For this review, take the finished solid that the model builds, in its own axes (mm). A direction names the side the tool comes from. Coordinates: 2 decimals unless noted, no trailing zeros. Return JSON: item names as keys, results as strings. Group by question number.
Item 1: For line 1 along X through (y, z) = (2, 4.5); line 2 along Y through (x, z) = (8.5, 15); line 3 along Y through (x, z) = (-28, 2.5), list the stretches that pass through material, from the lowest coordinate up.
Item 2: Machinability: for faces 1 (the flat face through (0, 1, 25)), 2 (the cylindrical face through (12.92, 1.24, 23.03)), which of the approach directions +Z, -Z, +X, -X, +Y, -Y give a long, thin tool a straight path to every point of the face, cutting with its end or side? Answer none if there is none.
Item 3: Draft analysis for pull direction Y (two halves, no side actions). For faces 3 (the flat face through (0, -52.325, 12)), 4 (the flat face through (0, 52.996, 12)), 5 (the flat face through (123.671, 0, 12)), 6 (the cylindrical face through (-52.47, 0.13, 12.33)), state which applies: +Y half, -Y half, draft (parallel to the pull), parting line (faces both ways), or undercut.
Item 4: Insertion check: pin 1 (13 mm diameter, centred on x = 8.98, y = 0, fed in from +Z); pin 2 (5.5 mm diameter, centred on x = -25.66, y = 0, fed in from +Z) (3 decimals); pin 3 (2.5 mm diameter, centred on x = 8, y = 1.5, fed in from +Z). Each pin has a flat end and moves straight along its axis. Give the tip position at first contact, or say it passes through.
```python
from build123d import *

# Parameters (mm, degrees)
F0_W           = 243.5423284769
F0_H           = 105.3215228021
F1_DEPTH       = 25
F3_D           = 6
F3_DEPTH       = 8
F3_TIP         = 1.8025818571
F4_D           = 6
F4_DEPTH       = 80
F4_TIP         = 1.8025818571
F5_D           = 6
F5_DEPTH       = 80
F5_CBORE_D     = 8.25
F5_CBORE_DEPTH = 4
F5_TIP         = 1.8025818571
F6_D           = 6
F6_DEPTH       = 10
F6_CBORE_D     = 8.25
F6_CBORE_DEPTH = 4
F6_TIP         = 1.8025818571
F7_D           = 6
F7_DEPTH       = 50
F7_CSINK_D     = 8.96
F7_CSINK_ANGLE = 90
F7_TIP         = 1.8025818571


with BuildPart() as f1:
    # F0 (on Top) → F1 (new body)
    with BuildSketch(Plane.XY):
        with Locations((1.9000694156, 0.3356132656)):
            Rectangle(F0_W, F0_H)
    extrude(amount=F1_DEPTH)

    # F3
    with Locations(Plane.XY.offset(25)):
        with Locations((-91.6707515717, 4.8113325611)):
            Hole(F3_D / 2, depth=F3_DEPTH)
            with Locations((0, 0, -(F3_DEPTH + F3_TIP / 2))):  # 118° drill point
                Cone(0, F3_D / 2, F3_TIP, mode=Mode.SUBTRACT)

    # F4
    with Locations(Plane.XY.offset(25)):
        with Locations((-55.4676242173, 0)):
            Hole(F4_D / 2, depth=F4_DEPTH)
            with Locations((0, 0, -(F4_DEPTH + F4_TIP / 2))):  # 118° drill point
                Cone(0, F4_D / 2, F4_TIP, mode=Mode.SUBTRACT)

    # F5
    with Locations(Plane.XY.offset(25)):
        with Locations((-25.6580132991, 0)):
            CounterBoreHole(F5_D / 2, F5_CBORE_D / 2, F5_CBORE_DEPTH, depth=F5_DEPTH)
            with Locations((0, 0, -(F5_DEPTH + F5_TIP / 2))):  # 118° drill point
                Cone(0, F5_D / 2, F5_TIP, mode=Mode.SUBTRACT)

    # F6
    with Locations(Plane.XY.offset(25)):
        with Locations((8.9849950746, 0)):
            CounterBoreHole(F6_D / 2, F6_CBORE_D / 2, F6_CBORE_DEPTH, depth=F6_DEPTH)
            with Locations((0, 0, -(F6_DEPTH + F6_TIP / 2))):  # 118° drill point
                Cone(0, F6_D / 2, F6_TIP, mode=Mode.SUBTRACT)

    # F7
    with Locations(Plane.XY.offset(25)):
        with Locations((33.6551889777, 0)):
            CounterSinkHole(F7_D / 2, F7_CSINK_D / 2, depth=F7_DEPTH, counter_sink_angle=F7_CSINK_ANGLE)
            with Locations((0, 0, -(F7_DEPTH + F7_TIP / 2))):  # 118° drill point
                Cone(0, F7_D / 2, F7_TIP, mode=Mode.SUBTRACT)


solid = f1.part
```
Findings below:
{
 "1": {"line 1": "x = -119.87 to -57.7, -53.23 to -27.89, -23.42 to 31.42, 35.89 to 123.67", "line 2": "y = -52.33 to -2.96, 2.96 to 53", "line 3": "y = -52.33 to -1.87, 1.87 to 53"},
 "2": {"face 1": "+Z, +X, -X, +Y, -Y", "face 2": "+Z"},
 "3": {"face 3": "-Y half", "face 4": "+Y half", "face 5": "draft", "face 6": "undercut"},
 "4": {"pin 1": "stops at z = 25", "pin 2": "passes through", "pin 3": "stops at z = 21"}
}
